Check sheet for the drawn part. Datum: minimum x, y, z corner. Units: mm. A direction names the side the tool comes from. Give positions to 0.01 mm unless a question says otherwise; leave off trailing zeros. Write each loop counter-clockwise with the first axis right and the second up, starting at its lowest first coordinate (ties: lowest second). Pieces come first, ordered by that corner, then holes. Notation, with made-up numbers: (52.5, 55) - (102.5, 55) arc R21 ccw to (102.5, 82) - close; hole circle Ø10 at (-36, 4.25). An arc over 180 degrees is marked (long way). Use a Markdown table: item, result.
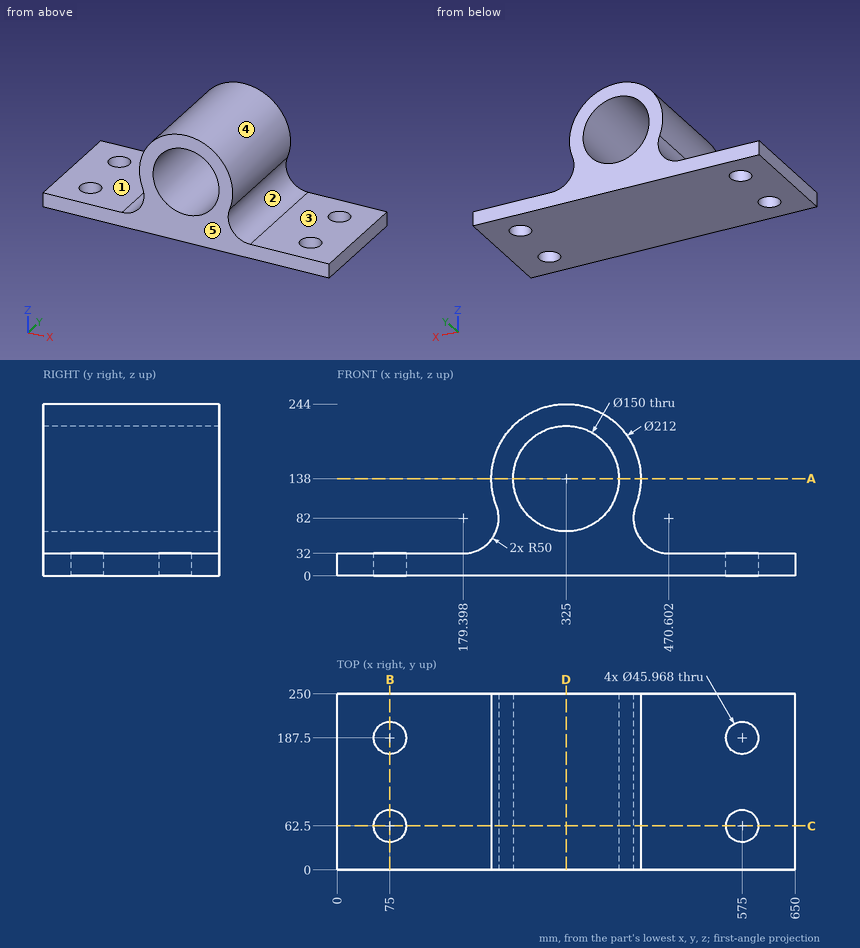
1) Section check A-A on z = 138. Record the boundary of the cut face in (x, y), then the cut area to 3 significant figures.
Working result:
| item | result |
|---|---|
| outline | (219, 0) - (250, 0) - (250, 250) - (219, 250) - close; (400, 0) - (431, 0) - (431, 250) - (400, 250) - close |
| area | 15,500 mm² |
2) Mould release check, pull along Z, two halves, no side actions. Record for the marked faces 3, 4 and 5: pulls with the +Z half, pulls with the -Z half, needs draft (parallel to the pull), parting line crosses it, or undercut.
Working result:
| item | result |
|---|---|
| face 3 | pulls with the +Z half |
| face 4 | undercut |
| face 5 | needs draft |
3) Section check D-D on x = 325. Record the boundary of the cut face in (y, z).
Working result:
| item | result |
|---|---|
| outline | (0, 0) - (250, 0) - (250, 63) - (0, 63) - close; (0, 213) - (250, 213) - (250, 244) - (0, 244) - close |
4) Depth check by flat-ended pin: P1, Ø1.5, axis at y = 201.5, z = 208, coming from the -X side; P2, Ø1, axis at y = 55.5, z = 107, coming from the +X side; P3, Ø6, axis at y = 160.5, z = 85, coming from the +X side. Enter the tip coordinate at first touch or a pass-through.
Working result:
| item | result |
|---|---|
| P1 | stops at x = 244.75 |
| P2 | stops at x = 426.52 |
| P3 | stops at x = 420.96 |
5) Section check B-B on x = 75. Record the boundary of the cut face in (y, z), then the cut area to 3 significant figures.
Working result:
| item | result |
|---|---|
| outline | (0, 0) - (39.52, 0) - (39.52, 32) - (0, 32) - close; (85.48, 0) - (164.52, 0) - (164.52, 32) - (85.48, 32) - close; (210.48, 0) - (250, 0) - (250, 32) - (210.48, 32) - close |
| area | 5,060 mm² |
6) Section check C-C on y = 62.5. Record the boundary of the cut face in (x, z) (1 decimal), then the cut area to 3 significant figures.
Working result:
| item | result |
|---|---|
| outline | (0, 0) - (52, 0) - (52, 32) - (0, 32) - close; (98, 0) - (552, 0) - (552, 32) - (470.6, 32) arc R50 cw to (423.9, 99.9) arc R106 ccw (long way) to (226.1, 99.9) arc R50 cw to (179.4, 32) - (98, 32) - close; (598, 0) - (650, 0) - (650, 32) - (598, 32) - close; hole circle Ø150 at (325, 138) |
| area | 39,800 mm² |
7) Set-up check for the marked faces 1 and 2: record each of +Z, -Z, +X, -X, +Y, -Y from which the full face is reachable in a straight line by a thin tool's end or side.
Working result:
| item | result |
|---|---|
| face 1 | +Z, -X, +Y, -Y |
| face 2 | +X, +Y, -Y |
8) Material ranges on L1, parallel to Y at x = 75, z = 25; L2, parallel to X at y = 62, z = 14; L3, parallel to Z at x = 38, y = 149.5, recorded low to high. Write a range as from..to.
Working result:
| item | result |
|---|---|
| L1 | y = 0..39.52, 85.48..164.52, 210.48..250 |
| L2 | x = 0..52.02, 97.98..552.02, 597.98..650 |
| L3 | z = 0..32 |
